Answer from the drawing. Dimensions are ordinates in mm from the lowest x, y and z of the part. Coordinates: 2 decimals unless noted, no trailing zeros. Order: outer loops, then holes, each group sorted by start corner. A loop starts at its lowest first (then second) coordinate and runs counter-clockwise, first axis right, second up. Notation, with made-up numbers: (-14, 75.25) -> (-7, 75.25) arc R30 cw to (-7, 110.25) -> close; hole circle Ø8 at (19, -35). An arc over 180 degrees is marked (long way). Answer in a Markdown table with one row per item.
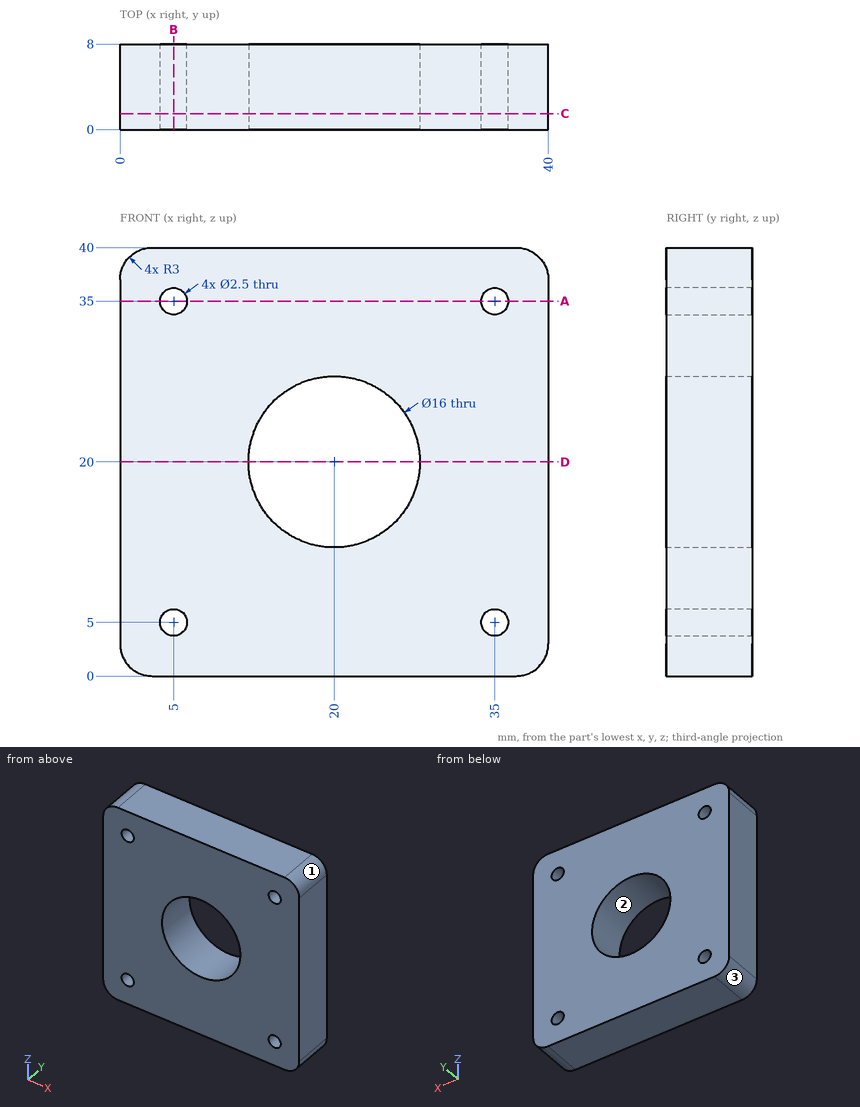
Q1. The part is cut by section D-D (z = 20). Write down the section's boundary in (x, y), then the cut area to 3 significant figures.
Outcome:
| item | result |
|---|---|
| outline | (0, 0) -> (12, 0) -> (12, 8) -> (0, 8) -> close; (28, 0) -> (40, 0) -> (40, 8) -> (28, 8) -> close |
| area | 192 mm² |
Q2. The part is cut by section C-C (y = 1.5). Write down the section's boundary in (x, z).
Outcome:
| item | result |
|---|---|
| outline | (0, 3) arc R3 ccw to (3, 0) -> (37, 0) arc R3 ccw to (40, 3) -> (40, 37) arc R3 ccw to (37, 40) -> (3, 40) arc R3 ccw to (0, 37) -> close; hole circle Ø2.5 at (5, 5); hole circle Ø2.5 at (5, 35); hole circle Ø16 at (20, 20); hole circle Ø2.5 at (35, 5); hole circle Ø2.5 at (35, 35) |
Q3. The part is cut by section A-A (z = 35). Write down the section's boundary in (x, y).
Outcome:
| item | result |
|---|---|
| outline | (0, 0) -> (3.75, 0) -> (3.75, 8) -> (0, 8) -> close; (6.25, 0) -> (33.75, 0) -> (33.75, 8) -> (6.25, 8) -> close; (36.25, 0) -> (40, 0) -> (40, 8) -> (36.25, 8) -> close |
Q4. Consider line 1 (X direction, y = 2, z = 35); line 2 (X direction, y = 4.75, z = 4); line 3 (X direction, y = 5, z = 20). Determine where each line is inside the solid, lowest interval first.
Outcome:
| item | result |
|---|---|
| line 1 | 0 to 3.75, 6.25 to 33.75, 36.25 to 40 |
| line 2 | 0 to 4.25, 5.75 to 34.25, 35.75 to 40 |
| line 3 | 0 to 12, 28 to 40 |
Q5. The part is cut by section B-B (x = 5). Write down the section's boundary in (y, z), then the cut area to 3 significant figures.
Outcome:
| item | result |
|---|---|
| outline | (0, 0) -> (8, 0) -> (8, 3.75) -> (0, 3.75) -> close; (0, 6.25) -> (8, 6.25) -> (8, 33.75) -> (0, 33.75) -> close; (0, 36.25) -> (8, 36.25) -> (8, 40) -> (0, 40) -> close |
| area | 280 mm² |
Q6. For a pull along X with two mould halves and no side action, classify the marked faces 1, 2 and 3 as pulls with the +X half, pulls with the -X half, needs draft (parallel to the pull), parting line crosses it, or undercut.
Outcome:
| item | result |
|---|---|
| face 1 | pulls with the +X half |
| face 2 | undercut |
| face 3 | pulls with the -X half |
